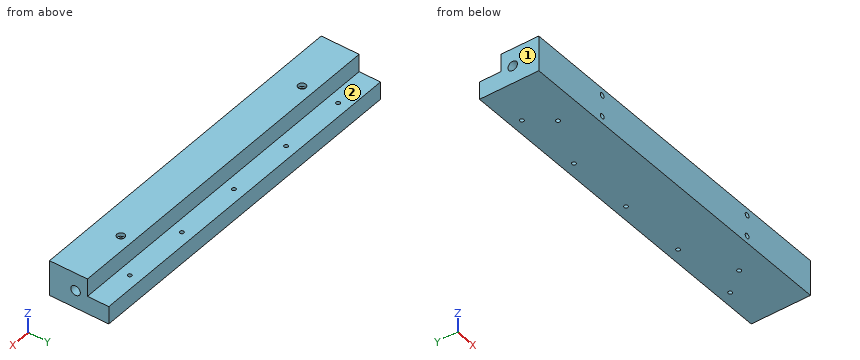
from build123d import *

# Parameters (mm, degrees)
SKETCH1_W                                       = 30
SKETCH1_H                                       = 32
BOSS_EXTRUDE1_DEPTH                             = 150
CUT_EXTRUDE1_REACH                              = 158.282
SKETCH2_W                                       = 15
SKETCH2_H                                       = 18
CUT_EXTRUDE1_DIRECTION_2_REACH                  = 158.282
CUT_EXTRUDE2_DEPTH                              = 161.934769394
CUT_EXTRUDE2_DEPTH_BACK                         = 161.934769394
SKETCH3_R                                       = 4
CBORE_FOR_M3_SOCKET_HEAD_CAP_SCREW1_D           = 3.4
CBORE_FOR_M3_SOCKET_HEAD_CAP_SCREW1_CBORE_D     = 6.5
CBORE_FOR_M3_SOCKET_HEAD_CAP_SCREW1_CBORE_DEPTH = 3
M4X0_7_TAPPED_HOLE1_D                           = 3.3
M5X0_8_TAPPED_HOLE1_D                           = 4.2
M5X0_8_TAPPED_HOLE1_DEPTH                       = 14
M5X0_8_TAPPED_HOLE1_TIP                         = 1.2618073


with BuildPart() as part:
    # Sketch1 → Boss-Extrude1 (new, symmetric)
    with BuildSketch(Plane(origin=(0, 0, 0), x_dir=(0, 0, -1), z_dir=(1, 0, 0))):
        with Locations((-15, 16)):
            Rectangle(SKETCH1_W, SKETCH1_H)
    extrude(amount=BOSS_EXTRUDE1_DEPTH, both=True)

    # Cut-Extrude1: up to this face of the body (flat: up to its plane)
    cut_extrude1_end = Plane(part.part.faces().sort_by_distance((150, 16, 15))[0])
    # Sketch2 → Cut-Extrude1 (add, up to the picked face)
    with BuildSketch(Plane(origin=(0, 0, 0), x_dir=(0, 0, -1), z_dir=(1, 0, 0)), mode=Mode.PRIVATE) as cut_extrude1_sk1:
        with Locations((-7.5, 41)):
            Rectangle(SKETCH2_W, SKETCH2_H)
    cut_extrude1_tool1 = split(extrude(cut_extrude1_sk1.sketch, amount=CUT_EXTRUDE1_REACH, mode=Mode.PRIVATE), bisect_by=cut_extrude1_end, keep=Keep.BOTH, mode=Mode.PRIVATE)
    add(cut_extrude1_tool1.solids().sort_by(Axis((0, 41, 7.5), (1, 0, 0)))[0])

    # Cut-Extrude1 direction 2: up to this face of the body (flat: up to its plane)
    cut_extrude1_direction_2_end = Plane(part.part.faces().sort_by_distance((-150, 16, 15))[0])
    # Sketch2 → Cut-Extrude1 direction 2 (add, up to the picked face)
    with BuildSketch(Plane(origin=(0, 0, 0), x_dir=(0, 0, -1), z_dir=(1, 0, 0)), mode=Mode.PRIVATE) as cut_extrude1_direction_2_sk1:
        with Locations((-7.5, 41)):
            Rectangle(SKETCH2_W, SKETCH2_H)
    cut_extrude1_direction_2_tool1 = split(extrude(cut_extrude1_direction_2_sk1.sketch, amount=-CUT_EXTRUDE1_DIRECTION_2_REACH, mode=Mode.PRIVATE), bisect_by=cut_extrude1_direction_2_end, keep=Keep.BOTH, mode=Mode.PRIVATE)
    add(cut_extrude1_direction_2_tool1.solids().sort_by(Axis((0, 41, 7.5), (-1, 0, 0)))[0])

    # Sketch3 → Cut-Extrude2 (cut, two sides: drawn at the far end of the back side and taken through both)
    with BuildSketch(Plane(origin=(0, 0, 0), x_dir=(0, 0, -1), z_dir=(1, 0, 0)).offset(-CUT_EXTRUDE2_DEPTH_BACK)):
        with Locations((-15, 22)):
            Circle(SKETCH3_R)
    extrude(amount=CUT_EXTRUDE2_DEPTH + CUT_EXTRUDE2_DEPTH_BACK, mode=Mode.SUBTRACT)

    # CBORE for M3 Socket Head Cap Screw1 (through all)
    with Locations(Plane.XY.offset(30)):
        with Locations((100, 22), (-100, 22)):
            CounterBoreHole(CBORE_FOR_M3_SOCKET_HEAD_CAP_SCREW1_D / 2, CBORE_FOR_M3_SOCKET_HEAD_CAP_SCREW1_CBORE_D / 2, CBORE_FOR_M3_SOCKET_HEAD_CAP_SCREW1_CBORE_DEPTH)

    # M4x0.7 Tapped Hole1 (through all)
    with Locations(Plane.XY.offset(15)):
        with Locations((115, 41), (57.5, 41), (0, 41), (-57.5, 41), (-115, 41)):
            Hole(M4X0_7_TAPPED_HOLE1_D / 2)

    # M5x0.8 Tapped Hole1
    with Locations(Plane.XZ):
        with Locations((-80, 24), (-80, 6), (80, 6), (80, 24)):
            Hole(M5X0_8_TAPPED_HOLE1_D / 2, depth=M5X0_8_TAPPED_HOLE1_DEPTH)
            with Locations((0, 0, -(M5X0_8_TAPPED_HOLE1_DEPTH + M5X0_8_TAPPED_HOLE1_TIP / 2))):  # 118° drill point
                Cone(0, M5X0_8_TAPPED_HOLE1_D / 2, M5X0_8_TAPPED_HOLE1_TIP, mode=Mode.SUBTRACT)


solid = part.part
Geometry check sheet. Reference: the model listing, model coordinates, mm. Face numbers are marked on the shaded views. A direction names the side the tool comes from. Coordinates: 2 decimals unless noted, no trailing zeros. Order: outer loops, then holes, each group sorted by start corner. A loop starts at its lowest first (then second) coordinate and runs counter-clockwise, first axis right, second up. Notation, with made-up numbers: (-18, -10.75) - (-4, -10.75) arc R23 cw to (-4, 13.25) - close; hole circle Ø10 at (-24, 67.5). An arc over 180 degrees is marked (long way). Answer in a Markdown table with one row per item. Add a question column.
1) Cross-section at B-B, the plane y = 35.5. Record the cut outline in (x, z), then the cut area to 3 significant figures.
2) Set-up check for the marked faces 1 and 2: record each of +Z, -Z, +X, -X, +Y, -Y from which the full face is reachable in a straight line by a thin tool's end or side.
3) Gauge pin test, flat ends, axial feed: P1, Ø10, axis at y = 38.5, z = 23.5, coming from the -X side; P2, Ø3, axis at x = -100, y = 21.5, coming from the +Z side; P3, Ø12, axis at x = -52.5, y = 42, coming from the +Z side; P4, Ø16.5, axis at x = 32.5, z = 25, coming from the +Y side. Record the tip position at first contact, or that the pin passes through.
4) Cross-section at A-A, the plane x = -88. Record the cut outline in (y, z), then the cut area to 3 significant figures.
5) Material ranges on line 1 along X through (y, z) = (22, 22.25); line 2 along X through (y, z) = (9, 6); line 3 along Y through (x, z) = (-115, 4.5), recorded low to high. Write a range as [from, to].
Check result:
| question | item | result |
|---|---|---|
| 1 | outline | (-150, 0) - (150, 0) - (150, 15) - (-150, 15) - close |
| 1 | area | 4,500 mm² |
| 2 | face 1 | +Z, -Z, -X, +Y, -Y |
| 2 | face 2 | +Z, +X, -X, +Y |
| 3 | P1 | passes through |
| 3 | P2 | stops at z = 27 |
| 3 | P3 | stops at z = 15 |
| 3 | P4 | stops at y = 32 |
| 4 | outline | (0, 0) - (50, 0) - (50, 15) - (32, 15) - (32, 30) - (0, 30) - close; hole circle Ø8 at (22, 15) |
| 4 | area | 1,180 mm² |
| 5 | line 1 | x = [-150, -101.7], [-98.3, 98.3], [101.7, 150] |
| 5 | line 2 | x = [-150, -82.1], [-77.9, 77.9], [82.1, 150] |
| 5 | line 3 | y = [0, 39.35], [42.65, 50] |
